Source: CAD feature listing. Evaluate the final solid. Frame: model axes, mm. Face numbers are marked on the shaded views. A direction names the side the tool comes from. Give positions to 0.01 mm unless a question says otherwise; leave off trailing zeros. Write each loop counter-clockwise with the first axis right and the second up, starting at its lowest first coordinate (ties: lowest second). Pieces come first, ordered by that corner, then holes. Notation, with made-up numbers: (-13.5, 46.5) -> (44.5, 46.5) arc R12 ccw to (44.5, 51.5) -> close; hole circle Ø2 at (30.5, 70.25). An arc over 180 degrees is marked (long way). Answer as a JSON object with one key per item and string values. Group by question number.
Item 1: Ray query, probe 1 along X at (y, z) = (64.5, -34.5); probe 2 along Z at (x, y) = (-47.5, 59); probe 3 along Z at (x, y) = (43, 26.5). Return the intervals inside material, ascending. Write a range as from..to.
Item 2: Pull-direction query (Z, two-part tool) for the marked faces 3, 4, 5 and 6; classes: pulls with the +Z half, pulls with the -Z half, needs draft (parallel to the pull), parting line crosses it, or undercut.
Item 3: First-contact query: pin 1 Ø5 at (x, z) = (-60, 48.5) entering from +Y; pin 2 Ø0.9 at (x, y) = (66, 66.5) entering from -Z; pin 3 Ø3.5 at (x, y) = (66.5, 69) entering from +Z. Flat tips, straight axial feed; report the tip coordinate or a pass-through.
Item 4: Section query B-B on x = 30.5. Return the cut outline in (y, z), plus the area to 3 significant figures.
Item 5: Section query C-C on z = 38.1. Give the number of separate pieces and of enclosed holes in the cut face, plus the area to 3 significant figures.
Item 6: Access query for the marked faces 1 and 2. Directions: +Z, -Z, +X, -X, +Y, -Y. A direction counts if a zero-diameter tool reaches every point of the face in a straight line with its end or side. Return the directions, or none.
Item 7: Section query D-D on x = 5.5. Return the cut outline in (y, z), plus the area to 3 significant figures.
from build123d import *

# Parameters (mm, degrees)
SKETCH2_W           = 135
SKETCH2_H           = 115
SKETCH2_W_2         = 126
SKETCH2_H_2         = 106
BOSS_EXTRUDE1_DEPTH = 70
SKETCH2_2_W         = 126
SKETCH2_2_H         = 106
BOSS_EXTRUDE2_DEPTH = 5
SKETCH3_W           = 121
SKETCH3_H           = 4.584314329
BOSS_EXTRUDE3_DEPTH = 4.5
SKETCH3_3_W         = 35
SKETCH3_3_H         = 12
CUT_EXTRUDE1_DEPTH  = 148.195448299
SKETCH11_W          = 69.2
SKETCH11_H          = 50
SKETCH11_R          = 2
CUT_EXTRUDE3_DEPTH  = 26.5
SKETCH21_R          = 5
CUT_EXTRUDE7_DEPTH  = 10
SKETCH12_W          = 4.5
SKETCH12_H          = 105.171400209
CUT_EXTRUDE4_DEPTH  = 5
SKETCH15_W          = 115
SKETCH15_H          = 70
CUT_EXTRUDE6_DEPTH  = 3
SKETCH17_W          = 120.925170316
SKETCH17_H          = 4.5
BOSS_EXTRUDE5_DEPTH = 5.5
FILLET1_R           = 3
FILLET2_R           = 3
FILLET3_R           = 3
SKETCH22_W          = 3
SKETCH22_H          = 105.171400209
BOSS_EXTRUDE8_DEPTH = 5
SKETCH14_W          = 19
SKETCH14_H          = 5
CUT_EXTRUDE5_DEPTH  = 5
SKETCH19_W          = 6.24417403
SKETCH19_H          = 4
BOSS_EXTRUDE6_DEPTH = 8
SKETCH20_W          = 4.447751713
SKETCH20_H          = 10.321902288
BOSS_EXTRUDE7_DEPTH = 8
FILLET5_R           = 3
FILLET6_R           = 3


# Some blends are built 0.0001 mm under size
with BuildPart() as part:
    # Sketch2 → Boss-Extrude1 (new body)
    with BuildSketch(Plane(origin=(0, 0, 0), x_dir=(1, 0, 0), z_dir=(0, 1, 0))):
        Rectangle(SKETCH2_W, SKETCH2_H)
        Rectangle(SKETCH2_W_2, SKETCH2_H_2, mode=Mode.SUBTRACT)
    extrude(amount=BOSS_EXTRUDE1_DEPTH)

    # Sketch2<2> → Boss-Extrude2 (add)
    with BuildSketch(Plane(origin=(0, 0, 0), x_dir=(1, 0, 0), z_dir=(0, 1, 0))):
        Rectangle(SKETCH2_2_W, SKETCH2_2_H)
    extrude(amount=BOSS_EXTRUDE2_DEPTH)

    # Sketch3 → Boss-Extrude3 (add)
    with BuildSketch(Plane.XY.offset(-53)):
        with Locations((0, 27.707842836)):
            Rectangle(SKETCH3_W, SKETCH3_H)
    extrude(amount=BOSS_EXTRUDE3_DEPTH)

    # Sketch3<3> → Cut-Extrude1 (cut, through all)
    with BuildSketch(Plane.XY.offset(-53)):
        with Locations((29, 37.5)):
            Rectangle(SKETCH3_3_W, SKETCH3_3_H)
    extrude(amount=-CUT_EXTRUDE1_DEPTH, mode=Mode.SUBTRACT)

    # Sketch11 → Cut-Extrude3 (cut)
    with BuildSketch(Plane.ZY.offset(67.5)):
        with Locations((-0.5, 30)):
            Rectangle(SKETCH11_W, SKETCH11_H)
        with BuildLine():
            ThreePointArc((39.9, 8.871779789), (36.1, 8), (39.9, 7.128220211))
            Line((39.9, 7.128220211), (39.9, 8.871779789))
        make_face()
        with BuildLine():
            Line((39.9, 51.128220211), (39.9, 52.871779789))
            ThreePointArc((39.9, 52.871779789), (36.1, 52), (39.9, 51.128220211))
        make_face()
        with Locations((-38.1, 52)):
            Circle(SKETCH11_R)
        with Locations((-38.1, 8)):
            Circle(SKETCH11_R)
    extrude(amount=-CUT_EXTRUDE3_DEPTH, mode=Mode.SUBTRACT)

    # Sketch21 → Cut-Extrude7 (cut)
    with BuildSketch(Plane(origin=(67.5, 0, 0), x_dir=(0, 0, -1), z_dir=(1, 0, 0))):
        with Locations((-26.20929228, 34.316365245)):
            Circle(SKETCH21_R)
    extrude(amount=-CUT_EXTRUDE7_DEPTH, mode=Mode.SUBTRACT)

    # Sketch12 → Cut-Extrude4 (cut)
    with BuildSketch(Plane(origin=(0, 70, 0), x_dir=(1, 0, 0), z_dir=(0, 1, 0))):
        with Locations((65.25, 0.414299895)):
            Rectangle(SKETCH12_W, SKETCH12_H)
    extrude(amount=-CUT_EXTRUDE4_DEPTH, mode=Mode.SUBTRACT)

    # Sketch15 → Cut-Extrude6 (cut)
    with BuildSketch(Plane.ZY.offset(67.5)):
        with Locations((0, 35)):
            Rectangle(SKETCH15_W, SKETCH15_H)
    extrude(amount=-CUT_EXTRUDE6_DEPTH, mode=Mode.SUBTRACT)

    # Sketch17 → Boss-Extrude5 (add)
    with BuildSketch(Plane(origin=(0, 0, 53), x_dir=(-1, 0, 0), z_dir=(0, 0, -1))):
        with Locations((0.074904723, 27.75)):
            Rectangle(SKETCH17_W, SKETCH17_H)
    extrude(amount=BOSS_EXTRUDE5_DEPTH)

    # Fillet1
    fillet1_edges = [part.edges().sort_by_distance(p)[0] for p in [
        (1.5, 0, 57.5),
        (1.5, 0, -57.5),
        (67.5, 0, 0),
    ]]
    fillet(fillet1_edges, radius=FILLET1_R)

    # Fillet2
    # the kernel refuses this fillet: 3 mm, written as the material it takes off along each edge
    with BuildSketch(Plane(origin=(64.5, 3, 54.5), x_dir=(0, 0, 1), z_dir=(1, 0, 0))) as fillet2_piece_1_section:
        Polygon((0, 0), (FILLET2_R, 0), (FILLET2_R, FILLET2_R), (0, FILLET2_R), align=None)
    fillet2_piece_1 = extrude(amount=FILLET2_R, mode=Mode.PRIVATE)
    fillet2_piece_1 = fillet2_piece_1 - Plane(origin=(64.5, 3, 54.5), x_dir=(0, 0.7071067811865475, -0.7071067811865475), z_dir=(1, 0, 0)) * Sphere(FILLET2_R, mode=Mode.PRIVATE)
    add(fillet2_piece_1, mode=Mode.SUBTRACT)
    with BuildSketch(Plane(origin=(64.5, 3, -54.5), x_dir=(1, 0, 0), z_dir=(0, 0, -1))) as fillet2_piece_2_section:
        Polygon((0, 0), (FILLET2_R, 0), (FILLET2_R, FILLET2_R), (0, FILLET2_R), align=None)
    fillet2_piece_2 = extrude(amount=FILLET2_R, mode=Mode.PRIVATE)
    fillet2_piece_2 = fillet2_piece_2 - Plane(origin=(64.5, 3, -54.5), x_dir=(-0.7071067811865475, 0.7071067811865475, 0), z_dir=(0, 0, -1)) * Sphere(FILLET2_R, mode=Mode.PRIVATE)
    add(fillet2_piece_2, mode=Mode.SUBTRACT)
    with BuildSketch(Plane(origin=(-64.5, 77.5, -57.5), x_dir=(1, 0, 0), z_dir=(0, -1, 0)), Plane(origin=(67.5, 3, 57.5), x_dir=(0, 0, -1), z_dir=(0, 1, 0)), Plane(origin=(67.5, 3, -57.5), x_dir=(-1, 0, 0), z_dir=(0, 1, 0))) as fillet2_piece_3:
        with BuildLine():
            CenterArc((FILLET2_R, FILLET2_R), FILLET2_R, 180, 90)
            Line((0, FILLET2_R), (0, 0))
            Line((0, 0), (FILLET2_R, 0))
        make_face()
    extrude(amount=74.5, mode=Mode.SUBTRACT)
    with BuildSketch(Plane(origin=(-64.5, 0, -54.5), x_dir=(0, 1, 0), z_dir=(0, 0, 1))) as fillet2_piece_4:
        with BuildLine():
            CenterArc((FILLET2_R, -FILLET2_R), FILLET2_R, 90, 90)
            Line((0, -FILLET2_R), (0, 0))
            Line((0, 0), (FILLET2_R, 0))
        make_face()
    extrude(amount=109, mode=Mode.SUBTRACT)
    with BuildSketch(Plane(origin=(-64.5, 3, 57.5), x_dir=(0, 0, -1), z_dir=(0, 1, 0))) as fillet2_piece_5:
        with BuildLine():
            CenterArc((FILLET2_R, -FILLET2_R), FILLET2_R, 90, 90)
            Line((0, -FILLET2_R), (0, 0))
            Line((0, 0), (FILLET2_R, 0))
        make_face()
    extrude(amount=74.5, mode=Mode.SUBTRACT)
    with BuildSketch(Plane(origin=(-64.5, 3, -54.5), x_dir=(0, 0, -1), z_dir=(0, 1, 0))) as fillet2_piece_6:
        with BuildLine():
            CenterArc((3 - FILLET2_R, -FILLET2_R), FILLET2_R, 0, 90)
            Line((3 - FILLET2_R, 0), (3, 0))
            Line((3, 0), (3, -FILLET2_R))
        make_face()
    revolve(axis=Axis((-64.5, 3, -54.5), (-1, 0, 0)), revolution_arc=90, mode=Mode.SUBTRACT)
    with BuildSketch(Plane(origin=(-64.5, 3, 54.5), x_dir=(0, -1, 0), z_dir=(0, 0, -1))) as fillet2_piece_7:
        with BuildLine():
            CenterArc((3 - FILLET2_R, -FILLET2_R), FILLET2_R, 360, 90)
            Line((3, -FILLET2_R), (3, 0))
            Line((3, 0), (3 - FILLET2_R, 0))
        make_face()
    revolve(axis=Axis((-64.5, 3, 54.5), (-1, 0, 0)), revolution_arc=90, mode=Mode.SUBTRACT)

    # Fillet3
    # the kernel refuses this fillet: 3 mm, written as the material it takes off along each edge
    with BuildSketch(Plane(origin=(67.5, 70, -54.5), x_dir=(-1, 0, 0), z_dir=(0, 0, 1))) as fillet3_piece_1:
        with BuildLine():
            CenterArc((FILLET3_R, FILLET3_R), FILLET3_R, 180, 90)
            Line((0, FILLET3_R), (0, 0))
            Line((0, 0), (FILLET3_R, 0))
        make_face()
    extrude(amount=9, mode=Mode.SUBTRACT)
    with BuildSketch(Plane(origin=(64.5, 70, -54.5), x_dir=(0, 0, -1), z_dir=(-1, 0, 0))) as fillet3_piece_2:
        with BuildLine():
            CenterArc((3 - FILLET3_R, FILLET3_R), FILLET3_R, 270, 90)
            Line((3 - FILLET3_R, 0), (3, 0))
            Line((3, 0), (3, FILLET3_R))
        make_face()
    revolve(axis=Axis((64.5, 70, -54.5), (0, -1, 0)), revolution_arc=90, mode=Mode.SUBTRACT)
    with BuildSketch(Plane(origin=(-61.5, 70, -57.5), x_dir=(0, -1, 0), z_dir=(1, 0, 0))) as fillet3_piece_3:
        with BuildLine():
            CenterArc((FILLET3_R, -FILLET3_R), FILLET3_R, 90, 90)
            Line((0, -FILLET3_R), (0, 0))
            Line((0, 0), (FILLET3_R, 0))
        make_face()
    extrude(amount=126, mode=Mode.SUBTRACT)
    with BuildSketch(Plane(origin=(-61.5, 70, -54.5), x_dir=(0, 0, -1), z_dir=(1, 0, 0))) as fillet3_piece_4:
        with BuildLine():
            CenterArc((3 - FILLET3_R, -FILLET3_R), FILLET3_R, 0, 90)
            Line((3, -FILLET3_R), (3, 0))
            Line((3, 0), (3 - FILLET3_R, 0))
        make_face()
    revolve(axis=Axis((-61.5, 70, -54.5), (0, 1, 0)), revolution_arc=90, mode=Mode.SUBTRACT)
    with BuildSketch(Plane(origin=(-64.5, 70, 54.5), x_dir=(1, 0, 0), z_dir=(0, 0, -1))) as fillet3_piece_5:
        with BuildLine():
            CenterArc((FILLET3_R, FILLET3_R), FILLET3_R, 180, 90)
            Line((0, FILLET3_R), (0, 0))
            Line((0, 0), (FILLET3_R, 0))
        make_face()
    extrude(amount=109, mode=Mode.SUBTRACT)
    with BuildSketch(Plane(origin=(-61.5, 70, 54.5), x_dir=(0, 0, 1), z_dir=(1, 0, 0))) as fillet3_piece_6:
        with BuildLine():
            CenterArc((3 - FILLET3_R, FILLET3_R), FILLET3_R, 270, 90)
            Line((3, FILLET3_R), (3, 0))
            Line((3, 0), (3 - FILLET3_R, 0))
        make_face()
    revolve(axis=Axis((-61.5, 70, 54.5), (0, -1, 0)), revolution_arc=90, mode=Mode.SUBTRACT)
    with BuildSketch(Plane(origin=(64.5, 70, 57.5), x_dir=(0, 0, -1), z_dir=(-1, 0, 0))) as fillet3_piece_7:
        with BuildLine():
            CenterArc((FILLET3_R, FILLET3_R), FILLET3_R, 180, 90)
            Line((0, FILLET3_R), (0, 0))
            Line((0, 0), (FILLET3_R, 0))
        make_face()
    extrude(amount=126, mode=Mode.SUBTRACT)
    with BuildSketch(Plane(origin=(64.5, 70, 54.5), x_dir=(1, 0, 0), z_dir=(0, 0, -1))) as fillet3_piece_8:
        with BuildLine():
            CenterArc((3 - FILLET3_R, FILLET3_R), FILLET3_R, 270, 90)
            Line((3, FILLET3_R), (3, 0))
            Line((3, 0), (3 - FILLET3_R, 0))
        make_face()
    revolve(axis=Axis((64.5, 70, 54.5), (0, -1, 0)), revolution_arc=90, mode=Mode.SUBTRACT)
    with BuildSketch(Plane(origin=(67.5, 70, 44.671400209), x_dir=(-1, 0, 0), z_dir=(0, 0, 1))) as fillet3_piece_9:
        with BuildLine():
            CenterArc((FILLET3_R, FILLET3_R), FILLET3_R, 180, 90)
            Line((0, FILLET3_R), (0, 0))
            Line((0, 0), (FILLET3_R, 0))
        make_face()
    extrude(amount=9.828599791, mode=Mode.SUBTRACT)

    # Sketch22 → Boss-Extrude8 (add)
    with BuildSketch(Plane(origin=(0, 65, 0), x_dir=(1, 0, 0), z_dir=(0, 1, 0))):
        with Locations((66, 0.414299895)):
            Rectangle(SKETCH22_W, SKETCH22_H)
    extrude(amount=BOSS_EXTRUDE8_DEPTH)

    # Sketch14 → Cut-Extrude5 (cut)
    with BuildSketch(Plane(origin=(67.5, 0, 0), x_dir=(0, 0, -1), z_dir=(1, 0, 0))):
        with Locations((-0.5, 67.5)):
            Rectangle(SKETCH14_W, SKETCH14_H)
    extrude(amount=-CUT_EXTRUDE5_DEPTH, mode=Mode.SUBTRACT)

    # Sketch19 → Boss-Extrude6 (add)
    with BuildSketch(Plane.XY.offset(-53)):
        with Locations((-59.877912985, 63.669872981)):
            Rectangle(SKETCH19_W, SKETCH19_H)
    extrude(amount=BOSS_EXTRUDE6_DEPTH)

    # Sketch20 → Boss-Extrude7 (add)
    with BuildSketch(Plane(origin=(0, 0, 53), x_dir=(-1, 0, 0), z_dir=(0, 0, -1))):
        with Locations((60.776124144, 60.508921837)):
            Rectangle(SKETCH20_W, SKETCH20_H)
    extrude(amount=BOSS_EXTRUDE7_DEPTH)

    # Fillet5
    fillet5_edges = [part.edges().sort_by_distance(p)[0] for p in [
        (67.5, 70, 31.085700105),
    ]]
    fillet(fillet5_edges, radius=FILLET5_R - 0.0001)  # a hair under: the kernel refuses the full size

    # Fillet6
    fillet6_edges = [part.edges().sort_by_distance(p)[0] for p in [
        (67.5, 70, -31),
    ]]
    fillet(fillet6_edges, radius=FILLET6_R - 0.0001)  # a hair under: the kernel refuses the full size


solid = part.part
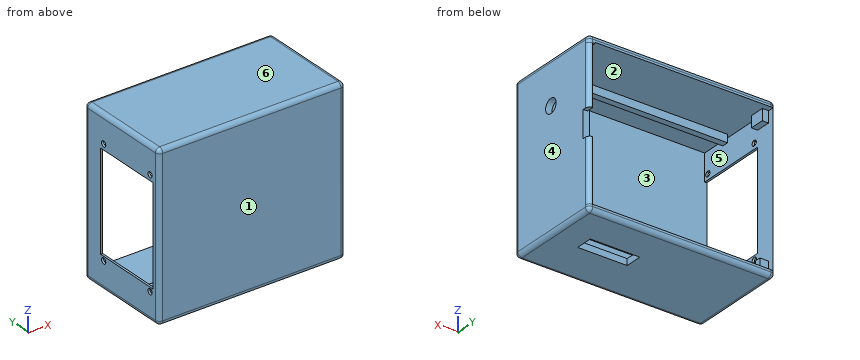
Worked answers:
{
 "1": {"probe 1": "-64.5..-63, 63..67.5", "probe 2": "-57.5..-53, 53..57.5", "probe 3": "-57.5..-48.5, 47.5..57.5"},
 "2": {"face 3": "undercut", "face 4": "needs draft", "face 5": "undercut", "face 6": "pulls with the +Z half"},
 "3": {"pin 1": "y = 65.67", "pin 2": "z = -57.31", "pin 3": "z = 57.3"},
 "4": {"outline": "(0, -54.5) arc R3 ccw to (3, -57.5) -> (31.5, -57.5) -> (31.5, -53) -> (30, -53) -> (30, -48.5) -> (25.42, -48.5) -> (25.42, -53) -> (5, -53) -> (5, 53) -> (25.5, 53) -> (25.5, 47.5) -> (30, 47.5) -> (30, 53) -> (70, 53) -> (70, 54.5) arc R3 ccw to (67, 57.5) -> (3, 57.5) arc R3 ccw to (0, 54.5) -> close; (43.5, -57.5) -> (67, -57.5) arc R3 ccw to (70, -54.5) -> (70, -53) -> (43.5, -53) -> close", "area": "1,140 mm^2"},
 "5": {"separate pieces": "3", "enclosed holes": "0", "area": "1,020 mm^2"},
 "6": {"face 1": "+Z, -Z, +X, -X, -Y", "face 2": "none"},
 "7": {"outline": "(0, -54.5) arc R3 ccw to (3, -57.5) -> (67, -57.5) arc R3 ccw to (70, -54.5) -> (70, -53) -> (30, -53) -> (30, -48.5) -> (25.42, -48.5) -> (25.42, -53) -> (5, -53) -> (5, 53) -> (25.5, 53) -> (25.5, 47.5) -> (30, 47.5) -> (30, 53) -> (70, 53) -> (70, 54.5) arc R3 ccw to (67, 57.5) -> (3, 57.5) arc R3 ccw to (0, 54.5) -> close", "area": "1,200 mm^2"}
}
